```python
from build123d import *

# Parameters (mm, degrees)
SKETCH_1_W               = 20
SKETCH_1_H               = 30
SKETCH_1_W_2             = 18
SKETCH_1_H_2             = 28
EXTRUDE_1_DEPTH          = 250
SKETCH_2_R               = 2.025
CUT_EXTRUDE_1_DEPTH      = 30
SKETCH_3_R               = 6
CUT_EXTRUDE_2_DEPTH      = 10
SKETCH_4_R               = 3
CUT_EXTRUDE_3_DEPTH      = 10
SKETCH_5_R               = 2.025
CUT_EXTRUDE_4_DEPTH      = 50
SKETCH_6_R               = 3.75
CUT_EXTRUDE_5_DEPTH      = 2
SKETCH_7_R               = 1.525
CUT_EXTRUDE_6_DEPTH      = 10
SKETCH_8_R               = 1.525
CUT_EXTRUDE_7_DEPTH      = 10
MIRROR_2_COPY_1_SKETCH_R = 1.525
MIRROR_2_COPY_1_DEPTH    = 10
MIRROR_2_COPY_2_SKETCH_R = 1.525
MIRROR_2_COPY_2_DEPTH    = 10
MIRROR_3_COPY_1_SKETCH_R = 1.525
MIRROR_3_COPY_1_DEPTH    = 10
MIRROR_3_COPY_2_SKETCH_R = 1.525
MIRROR_3_COPY_2_DEPTH    = 10
MIRROR_3_COPY_3_SKETCH_R = 1.525
MIRROR_3_COPY_3_DEPTH    = 10
MIRROR_3_COPY_4_SKETCH_R = 1.525
MIRROR_3_COPY_4_DEPTH    = 10
MIRROR_3_COPY_5_SKETCH_R = 1.525
MIRROR_3_COPY_5_DEPTH    = 10
MIRROR_3_COPY_6_SKETCH_R = 1.525
MIRROR_3_COPY_6_DEPTH    = 10
CUT_EXTRUDE_8_DEPTH      = 10
SKETCH_11_R              = 2.475
CUT_EXTRUDE_9_DEPTH      = 10
SKETCH_12_R              = 2.025
CUT_EXTRUDE_10_DEPTH     = 20


with BuildPart() as part:
    # Sketch 1 → Extrude 1 (new body, symmetric)
    with BuildSketch(Plane.XY):
        Rectangle(SKETCH_1_W, SKETCH_1_H)
        Rectangle(SKETCH_1_W_2, SKETCH_1_H_2, mode=Mode.SUBTRACT)
    extrude(amount=EXTRUDE_1_DEPTH, both=True)

    # Sketch 2 → Cut-Extrude 1 (cut)
    with BuildSketch(Plane(origin=(0, 15, 0), x_dir=(1, 0, 0), z_dir=(0, 1, 0))):
        with Locations((0, -240)):
            Circle(SKETCH_2_R)
        with Locations((0, -220)):
            Circle(SKETCH_2_R)
        with Locations((0, 240)):
            Circle(SKETCH_2_R)
        with Locations((0, 220)):
            Circle(SKETCH_2_R)
    extrude(amount=-CUT_EXTRUDE_1_DEPTH, mode=Mode.SUBTRACT)

    # Sketch 3 → Cut-Extrude 2 (cut)
    with BuildSketch(Plane.XZ.offset(15)):
        Circle(SKETCH_3_R)
    extrude(amount=-CUT_EXTRUDE_2_DEPTH, mode=Mode.SUBTRACT)

    # Sketch 4 → Cut-Extrude 3 (cut)
    with BuildSketch(Plane.XZ.offset(-14)):
        Circle(SKETCH_4_R)
    extrude(amount=-CUT_EXTRUDE_3_DEPTH, mode=Mode.SUBTRACT)

    # Sketch 5 → Cut-Extrude 4 (cut)
    with BuildSketch(Plane.XZ.offset(15)):
        with Locations((0, 56)):
            Circle(SKETCH_5_R)
        with Locations((0, 74)):
            Circle(SKETCH_5_R)
        with Locations((0, -74)):
            Circle(SKETCH_5_R)
        with Locations((0, -56)):
            Circle(SKETCH_5_R)
    extrude(amount=-CUT_EXTRUDE_4_DEPTH, mode=Mode.SUBTRACT)

    # Sketch 6 → Cut-Extrude 5 (cut)
    with BuildSketch(Plane.XZ.offset(15)):
        with Locations((0, 74)):
            Circle(SKETCH_6_R)
        with Locations((0, 56)):
            Circle(SKETCH_6_R)
        with Locations((0, -56)):
            Circle(SKETCH_6_R)
        with Locations((0, -74)):
            Circle(SKETCH_6_R)
    extrude(amount=-CUT_EXTRUDE_5_DEPTH, mode=Mode.SUBTRACT)

    # Sketch 7 → Cut-Extrude 6 (cut)
    with BuildSketch(Plane(origin=(0, 15, 0), x_dir=(1, 0, 0), z_dir=(0, 1, 0))):
        with Locations((6, 115)):
            Circle(SKETCH_7_R)
        with Locations((6, 95)):
            Circle(SKETCH_7_R)
        with Locations((6, 150)):
            Circle(SKETCH_7_R)
        with Locations((6, 170)):
            Circle(SKETCH_7_R)
    cut_extrude_6 = extrude(amount=-CUT_EXTRUDE_6_DEPTH, mode=Mode.SUBTRACT)

    # Sketch 8 → Cut-Extrude 7 (cut)
    with BuildSketch(Plane(origin=(10, 0, 0), x_dir=(0, 0, -1), z_dir=(1, 0, 0))):
        with Locations((105, 11)):
            Circle(SKETCH_8_R)
        with Locations((125, 11)):
            Circle(SKETCH_8_R)
        with Locations((160, 11)):
            Circle(SKETCH_8_R)
        with Locations((180, 11)):
            Circle(SKETCH_8_R)
    cut_extrude_7 = extrude(amount=-CUT_EXTRUDE_7_DEPTH, mode=Mode.SUBTRACT)

    # Mirror 1: Cut-Extrude 6, Cut-Extrude 7 across plane
    add(cut_extrude_6.mirror(Plane.ZX), mode=Mode.SUBTRACT)
    add(cut_extrude_7.mirror(Plane.ZX), mode=Mode.SUBTRACT)

    # Mirror 2: Cut-Extrude 6, Cut-Extrude 7 across plane
    add(cut_extrude_6.mirror(Plane.XY), mode=Mode.SUBTRACT)
    add(cut_extrude_7.mirror(Plane.XY), mode=Mode.SUBTRACT)

    # Mirror 2 copy 1 sketch → Mirror 2 copy 1 (cut)
    with BuildSketch(Plane.XZ.offset(15)):
        with Locations((6, 115)):
            Circle(MIRROR_2_COPY_1_SKETCH_R)
        with Locations((6, 95)):
            Circle(MIRROR_2_COPY_1_SKETCH_R)
        with Locations((6, 150)):
            Circle(MIRROR_2_COPY_1_SKETCH_R)
        with Locations((6, 170)):
            Circle(MIRROR_2_COPY_1_SKETCH_R)
    extrude(amount=-MIRROR_2_COPY_1_DEPTH, mode=Mode.SUBTRACT)

    # Mirror 2 copy 2 sketch → Mirror 2 copy 2 (cut)
    with BuildSketch(Plane(origin=(10, 0, 0), x_dir=(0, 0, 1), z_dir=(1, 0, 0))):
        with Locations((105, 11)):
            Circle(MIRROR_2_COPY_2_SKETCH_R)
        with Locations((125, 11)):
            Circle(MIRROR_2_COPY_2_SKETCH_R)
        with Locations((160, 11)):
            Circle(MIRROR_2_COPY_2_SKETCH_R)
        with Locations((180, 11)):
            Circle(MIRROR_2_COPY_2_SKETCH_R)
    extrude(amount=-MIRROR_2_COPY_2_DEPTH, mode=Mode.SUBTRACT)

    # Mirror 3: Cut-Extrude 6, Cut-Extrude 7 across plane
    add(cut_extrude_6.mirror(Plane(origin=(0, 0, 0), x_dir=(0, 0, 1), z_dir=(1, 0, 0))), mode=Mode.SUBTRACT)
    add(cut_extrude_7.mirror(Plane(origin=(0, 0, 0), x_dir=(0, 0, 1), z_dir=(1, 0, 0))), mode=Mode.SUBTRACT)

    # Mirror 3 copy 1 sketch → Mirror 3 copy 1 (cut)
    with BuildSketch(Plane(origin=(0, 15, 0), x_dir=(-1, 0, 0), z_dir=(0, 1, 0))):
        with Locations((6, 115)):
            Circle(MIRROR_3_COPY_1_SKETCH_R)
        with Locations((6, 95)):
            Circle(MIRROR_3_COPY_1_SKETCH_R)
        with Locations((6, 150)):
            Circle(MIRROR_3_COPY_1_SKETCH_R)
        with Locations((6, 170)):
            Circle(MIRROR_3_COPY_1_SKETCH_R)
    extrude(amount=-MIRROR_3_COPY_1_DEPTH, mode=Mode.SUBTRACT)

    # Mirror 3 copy 2 sketch → Mirror 3 copy 2 (cut)
    with BuildSketch(Plane.ZY.offset(10)):
        with Locations((105, 11)):
            Circle(MIRROR_3_COPY_2_SKETCH_R)
        with Locations((125, 11)):
            Circle(MIRROR_3_COPY_2_SKETCH_R)
        with Locations((160, 11)):
            Circle(MIRROR_3_COPY_2_SKETCH_R)
        with Locations((180, 11)):
            Circle(MIRROR_3_COPY_2_SKETCH_R)
    extrude(amount=-MIRROR_3_COPY_2_DEPTH, mode=Mode.SUBTRACT)

    # Mirror 3 copy 3 sketch → Mirror 3 copy 3 (cut)
    with BuildSketch(Plane(origin=(0, -15, 0), x_dir=(-1, 0, 0), z_dir=(0, -1, 0))):
        with Locations((6, -115)):
            Circle(MIRROR_3_COPY_3_SKETCH_R)
        with Locations((6, -95)):
            Circle(MIRROR_3_COPY_3_SKETCH_R)
        with Locations((6, -150)):
            Circle(MIRROR_3_COPY_3_SKETCH_R)
        with Locations((6, -170)):
            Circle(MIRROR_3_COPY_3_SKETCH_R)
    extrude(amount=-MIRROR_3_COPY_3_DEPTH, mode=Mode.SUBTRACT)

    # Mirror 3 copy 4 sketch → Mirror 3 copy 4 (cut)
    with BuildSketch(Plane.ZY.offset(10)):
        with Locations((105, -11)):
            Circle(MIRROR_3_COPY_4_SKETCH_R)
        with Locations((125, -11)):
            Circle(MIRROR_3_COPY_4_SKETCH_R)
        with Locations((160, -11)):
            Circle(MIRROR_3_COPY_4_SKETCH_R)
        with Locations((180, -11)):
            Circle(MIRROR_3_COPY_4_SKETCH_R)
    extrude(amount=-MIRROR_3_COPY_4_DEPTH, mode=Mode.SUBTRACT)

    # Mirror 3 copy 5 sketch → Mirror 3 copy 5 (cut)
    with BuildSketch(Plane(origin=(0, -15, 0), x_dir=(-1, 0, 0), z_dir=(0, -1, 0))):
        with Locations((6, 115)):
            Circle(MIRROR_3_COPY_5_SKETCH_R)
        with Locations((6, 95)):
            Circle(MIRROR_3_COPY_5_SKETCH_R)
        with Locations((6, 150)):
            Circle(MIRROR_3_COPY_5_SKETCH_R)
        with Locations((6, 170)):
            Circle(MIRROR_3_COPY_5_SKETCH_R)
    extrude(amount=-MIRROR_3_COPY_5_DEPTH, mode=Mode.SUBTRACT)

    # Mirror 3 copy 6 sketch → Mirror 3 copy 6 (cut)
    with BuildSketch(Plane(origin=(-10, 0, 0), x_dir=(0, 0, -1), z_dir=(-1, 0, 0))):
        with Locations((105, 11)):
            Circle(MIRROR_3_COPY_6_SKETCH_R)
        with Locations((125, 11)):
            Circle(MIRROR_3_COPY_6_SKETCH_R)
        with Locations((160, 11)):
            Circle(MIRROR_3_COPY_6_SKETCH_R)
        with Locations((180, 11)):
            Circle(MIRROR_3_COPY_6_SKETCH_R)
    extrude(amount=-MIRROR_3_COPY_6_DEPTH, mode=Mode.SUBTRACT)

    # Sketch 9 → Cut-Extrude 8 (cut)
    with BuildSketch(Plane.XZ.offset(15)):
        with BuildLine():
            Line((6, 12.5), (6, -12.5))
            ThreePointArc((6, -12.5), (0, -18.5), (-6, -12.5))
            Line((-6, -12.5), (-6, 12.5))
            ThreePointArc((-6, 12.5), (0, 18.5), (6, 12.5))
        make_face()
    extrude(amount=-CUT_EXTRUDE_8_DEPTH, mode=Mode.SUBTRACT)

    # Sketch 11 → Cut-Extrude 9 (cut)
    with BuildSketch(Plane.XZ.offset(15)):
        with Locations((0, 25)):
            Circle(SKETCH_11_R)
        with Locations((0, -25)):
            Circle(SKETCH_11_R)
    extrude(amount=-CUT_EXTRUDE_9_DEPTH, mode=Mode.SUBTRACT)

    # Sketch 12 → Cut-Extrude 10 (cut)
    with BuildSketch(Plane(origin=(10, 0, 0), x_dir=(0, 0, -1), z_dir=(1, 0, 0))):
        with Locations((-232, 5)):
            Circle(SKETCH_12_R)
        with Locations((-232, -5)):
            Circle(SKETCH_12_R)
        with Locations((232, -5)):
            Circle(SKETCH_12_R)
        with Locations((232, 5)):
            Circle(SKETCH_12_R)
    extrude(amount=-CUT_EXTRUDE_10_DEPTH, mode=Mode.SUBTRACT)


solid = part.part
```
Geometry check sheet. Reference: the model listing, model coordinates, mm. A direction names the side the tool comes from. Give positions to 0.01 mm unless a question says otherwise; leave off trailing zeros. Order: outer loops, then holes, each group sorted by start corner. A loop starts at its lowest first (then second) coordinate and runs counter-clockwise, first axis right, second up.
1. Section check A-A, the plane z = 33.5. Enter the section's corners in (x, y), and give its area (3 significant figures).
2. Access from +Z, -Z, +X, -X, +Y, -Y to the whole of each face (thin tool, end or side, straight path). Record for faces 5 (the face through (-8, -14, 4)), 6 (the face through (-9.7, 0.1, -250)).
3. Gauge pin test, flat ends, axial feed: pin 1 Ø2.5 at (x, z) = (6, 150) entering from +Y (1 decimal); pin 2 Ø3 at (x, z) = (0, -25) entering from -Y. Record the tip position at first contact, or that the pin passes through.
4. Thickness scan on L1, parallel to X at y = -14.8, z = 150 (3 decimals); L2, parallel to Y at x = 9.4, z = -232 (3 decimals); L3, parallel to X at y = 8, z = 140.5. Record the ranges inside material, lowest first.
5. Release check for a two-part mould opening along X. For faces 1 (the face through (-9, 0, 4)), 2 (the face through (10, 0, 4)), 3 (the face through (9, 0, 4)), 4 (the face through (0, 15, 4)) record: pulls with the +X half, pulls with the -X half, needs draft (parallel to the pull), parting line crosses it, or undercut.
Values follow:
1. outline: (-10, -15) - (10, -15) - (10, 15) - (-10, 15) - close; hole (-9, -14) - (9, -14) - (9, 14) - (-9, 14) - close
1. area: 96.0 mm2
2. face 5: +Z, -Z
2. face 6: -Z, +X, -X, +Y, -Y
3. pin 1: passes through
3. pin 2: stops at y = 14
4. L1: x = -10 to -7.525, -4.475 to 4.475, 7.525 to 10
4. L2: y = -15 to -7.025, -2.975 to 2.975, 7.025 to 15
4. L3: x = -10 to -9, 9 to 10
5. face 1: undercut
5. face 2: pulls with the +X half
5. face 3: undercut
5. face 4: needs draft
